Part model, mm, in its own coordinate system. A direction names the side the tool comes from. Round coordinates to 2 decimals unless told otherwise and drop trailing zeros. Return JSON: item names as keys, results as strings. Group by question number.
```python
from build123d import *

# Parameters (mm, degrees)
BOSS_EXTRUDE1_DEPTH     = 105
CUT_EXTRUDE1_DEPTH      = 105.1
CUT_EXTRUDE1_DEPTH_BACK = 105.1
SKETCH4_W               = 78.145475997
SKETCH4_H               = 46.57
SKETCH5_W               = 111.656527507
SKETCH5_H               = 70.51
SKETCH8_R               = 23.092737718
SKETCH8_R_2             = 19.459118311
CUT_EXTRUDE4_DEPTH      = 40.5550001
CUT_EXTRUDE4_DEPTH_BACK = 40.5550001
SKETCH9_R               = 16.617220832
SKETCH9_R_2             = 16.520725145
SKETCH9_R_3             = 19.698995854
CUT_EXTRUDE5_DEPTH      = 40.5550001
CUT_EXTRUDE5_DEPTH_BACK = 40.5550001


with BuildPart() as part:
    # Sketch1 → Boss-Extrude1 (new body)
    with BuildSketch(Plane.XY):
        Polygon((0, 39.555), (0, -39.555), (326.3, -27.585), (326.3, 27.585), align=None)
    extrude(amount=BOSS_EXTRUDE1_DEPTH)

    # Sketch3 → Cut-Extrude1 (cut, two sides)
    with BuildSketch(Plane(origin=(0, 0, 0), x_dir=(1, 0, 0), z_dir=(0, 1, 0))) as cut_extrude1_sk:
        Polygon((0, -15), (84.7, -25.82), (154.7, -25.82), (326.3, -54.6), (326.3, 36.079011671), (0, 41.113860107), align=None)
    extrude(amount=CUT_EXTRUDE1_DEPTH, mode=Mode.SUBTRACT)
    extrude(cut_extrude1_sk.sketch, amount=-CUT_EXTRUDE1_DEPTH_BACK, mode=Mode.SUBTRACT)

    # Sketch4 → Cut-Loft1 section 0
    with BuildSketch(Plane(origin=(326.3, 0, 0), x_dir=(0, 0, -1), z_dir=(1, 0, 0))):
        with Locations((-61.627262002, 0)):
            Rectangle(SKETCH4_W, SKETCH4_H)
    # Sketch5 → Cut-Loft1 section 1
    with BuildSketch(Plane.ZY):
        with Locations((44.871736246, 0)):
            Rectangle(SKETCH5_W, SKETCH5_H)
    loft(mode=Mode.SUBTRACT)

    # Sketch8 → Cut-Extrude4 (cut, two sides)
    with BuildSketch(Plane(origin=(0, 0, 0), x_dir=(1, 0, 0), z_dir=(0, 1, 0))) as cut_extrude4_sk:
        with Locations((214.641912664, -70.440417493)):
            Circle(SKETCH8_R)
        with Locations((278.393804533, -73.204497515)):
            Circle(SKETCH8_R_2)
    extrude(amount=CUT_EXTRUDE4_DEPTH, mode=Mode.SUBTRACT)
    extrude(cut_extrude4_sk.sketch, amount=-CUT_EXTRUDE4_DEPTH_BACK, mode=Mode.SUBTRACT)

    # Sketch9 → Cut-Extrude5 (cut, two sides)
    with BuildSketch(Plane(origin=(0, 0, 0), x_dir=(1, 0, 0), z_dir=(0, 1, 0))) as cut_extrude5_sk:
        with Locations((118.110707971, -47.394014977)):
            Circle(SKETCH9_R)
        with Locations((72.426153878, -47.394014977)):
            Circle(SKETCH9_R_2)
        with Locations((164.053366889, -60.04115142)):
            Circle(SKETCH9_R_3)
        Polygon((4.3, -6.491738735), (44.3, -6.491738735), (44.3, -68.95), (136.3, -68.95), (136.3, -100.7), (44.3, -100.7), (4.3, -100.7), align=None)
    extrude(amount=CUT_EXTRUDE5_DEPTH, mode=Mode.SUBTRACT)
    extrude(cut_extrude5_sk.sketch, amount=-CUT_EXTRUDE5_DEPTH_BACK, mode=Mode.SUBTRACT)


solid = part.part
```
Item 1: Wall check: L1, parallel to Y at x = 136.5, z = 81.5; L2, parallel to Z at x = 148, y = -20.5; L3, parallel to Y at x = 143.5, z = 55.5. Give the ranges that are in metal, low to high.
Item 2: Flat gauge pins, fed straight in: P1, Ø2, axis at y = -33.5, z = 85, coming from the -X side; P2, Ø3.5, axis at x = 132.5, y = 33.5, coming from the -Z side; P3, Ø3.5, axis at y = -36.5, z = 41, coming from the +X side; P4, Ø2, axis at y = 36, z = 49, coming from the -X side. Where does each tip first touch, or does it go through?
Item 3: Cut at A-A (x = 285.5). State how many separate pieces and enclosed holes the cut face has, then the cut area to 3 significant figures.
Item 4: Two-plate mould, pull along X, no slides. Class faces 4 (the face through (186.56, -32.71, 73.12)), 5 (the face through (114.508, -33.062, 63.616)), 6 (the face through (90, -34, 68.95)): released by +X, released by -X, zero draft, split by the parting line, or undercut.
Item 5: Which spindle directions (+Z, -Z, +X, -X, +Y, -Y) get a long thin tool onto all of the face, cutting with end or side? Do faces 1 (the face through (119, -33, 25.82)), 2 (the face through (188.082, 32.655, 66.457)), 3 (the face through (69, 35, 100.7)). Say none if no direction does.
Checks:
{
 "1": {"L1": "y = -34.55 to -30.25, 30.25 to 34.55", "L2": "z = 100.7 to 105", "L3": "y = -34.29 to -29.99, 29.99 to 34.29"},
 "2": {"P1": "stops at x = 136.3", "P2": "stops at z = 25.82", "P3": "stops at x = 103.53", "P4": "stops at x = 0"},
 "3": {"separate pieces": "3", "enclosed holes": "0", "area": "394 mm2"},
 "4": {"face 4": "released by +X", "face 5": "undercut", "face 6": "zero draft"},
 "5": {"face 1": "-Z, +X, +Y, -Y", "face 2": "+Z, -Z, +X, +Y", "face 3": "+Y, -Y"}
}
